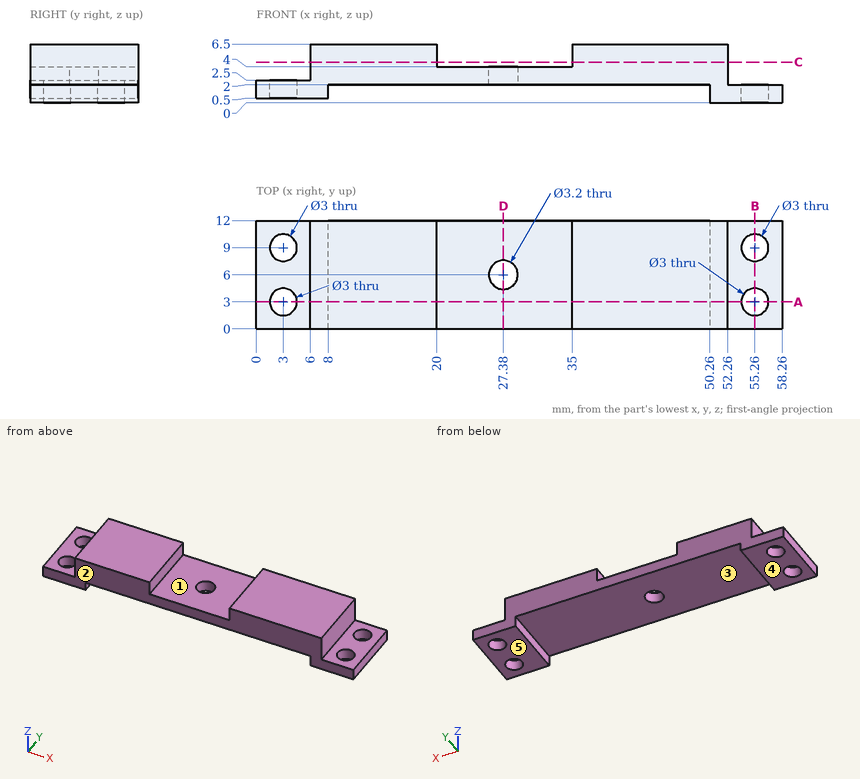
Geometry: see drawing. Coordinates: mm, zero at the bounding-box minimum. A direction names the side the tool comes from. Coordinates: 2 decimals unless noted, no trailing zeros. Order: outer loops, then holes, each group sorted by start corner. A loop starts at its lowest first (then second) coordinate and runs counter-clockwise, first axis right, second up. Notation, with made-up numbers: (9, -40) -> (40, -40) arc R22 ccw to (40, -31) -> close; hole circle Ø1 at (-31.75, 41). An arc over 180 degrees is marked (long way). Write each question's results on one line, items separated by ' | '. Start each with the question number.
1) Cut plane B-B, the plane x = 55.26. Output: boundary loops of the cut face in (y, z).
2) Cut plane D-D, the plane x = 27.38. Output: boundary loops of the cut face in (y, z).
3) Cut plane A-A, the plane y = 3. Output: boundary loops of the cut face in (x, z).
4) Mould query, pull axis X, two halves, no side actions, for the marked faces 1 and 2. Classes: released by +X, released by -X, zero draft, split by the parting line, or undercut.
5) Material intervals for line 1 along Y through (x, z) = (3, 2); line 2 along X through (y, z) = (7.5, 4.75); line 3 along X through (y, z) = (5.75, 1), sorted ascending.
6) Cut plane C-C, the plane z = 4.5. Output: boundary loops of the cut face in (x, y).
7) Set-up query: the marked faces 3, 4 and 5. Return all of +Z, -Z, +X, -X, +Y, -Y with unobstructed straight access to the full face (end or side cutting, diameter ignored); none if empty.
8) First-contact query: pin 1 (0.8 mm diameter, centred on y = 4.5, z = 5.5, fed in from -X); pin 2 (3 mm diameter, centred on y = 8, z = 5.5, fed in from +X); pin 3 (3.5 mm diameter, centred on x = 23, y = 6, fed in from -Z). Flat tips, straight axial feed; report the tip coordinate or a pass-through.
Checks:
1) outline: (0, 0) -> (1.5, 0) -> (1.5, 2) -> (0, 2) -> close; (4.5, 0) -> (7.5, 0) -> (7.5, 2) -> (4.5, 2) -> close; (10.5, 0) -> (12, 0) -> (12, 2) -> (10.5, 2) -> close
2) outline: (0, 2) -> (4.4, 2) -> (4.4, 4) -> (0, 4) -> close; (7.6, 2) -> (12, 2) -> (12, 4) -> (7.6, 4) -> close
3) outline: (0, 0.5) -> (1.5, 0.5) -> (1.5, 2.5) -> (0, 2.5) -> close; (4.5, 0.5) -> (8, 0.5) -> (8, 2) -> (50.26, 2) -> (50.26, 0) -> (53.76, 0) -> (53.76, 2) -> (52.26, 2) -> (52.26, 6.5) -> (35, 6.5) -> (35, 4) -> (20, 4) -> (20, 6.5) -> (6, 6.5) -> (6, 2.5) -> (4.5, 2.5) -> close; (56.76, 0) -> (58.26, 0) -> (58.26, 2) -> (56.76, 2) -> close
4) face 1: undercut | face 2: zero draft
5) line 1: 0 to 1.5, 4.5 to 7.5, 10.5 to 12 | line 2: 6 to 20, 35 to 52.26 | line 3: 0 to 8, 50.26 to 58.26
6) outline: (6, 0) -> (20, 0) -> (20, 12) -> (6, 12) -> close; (35, 0) -> (52.26, 0) -> (52.26, 12) -> (35, 12) -> close
7) face 3: -Z, +Y, -Y | face 4: -Z, -X, +Y, -Y | face 5: -Z, +X, -X, +Y, -Y
8) pin 1: x = 6 | pin 2: x = 52.26 | pin 3: z = 2
